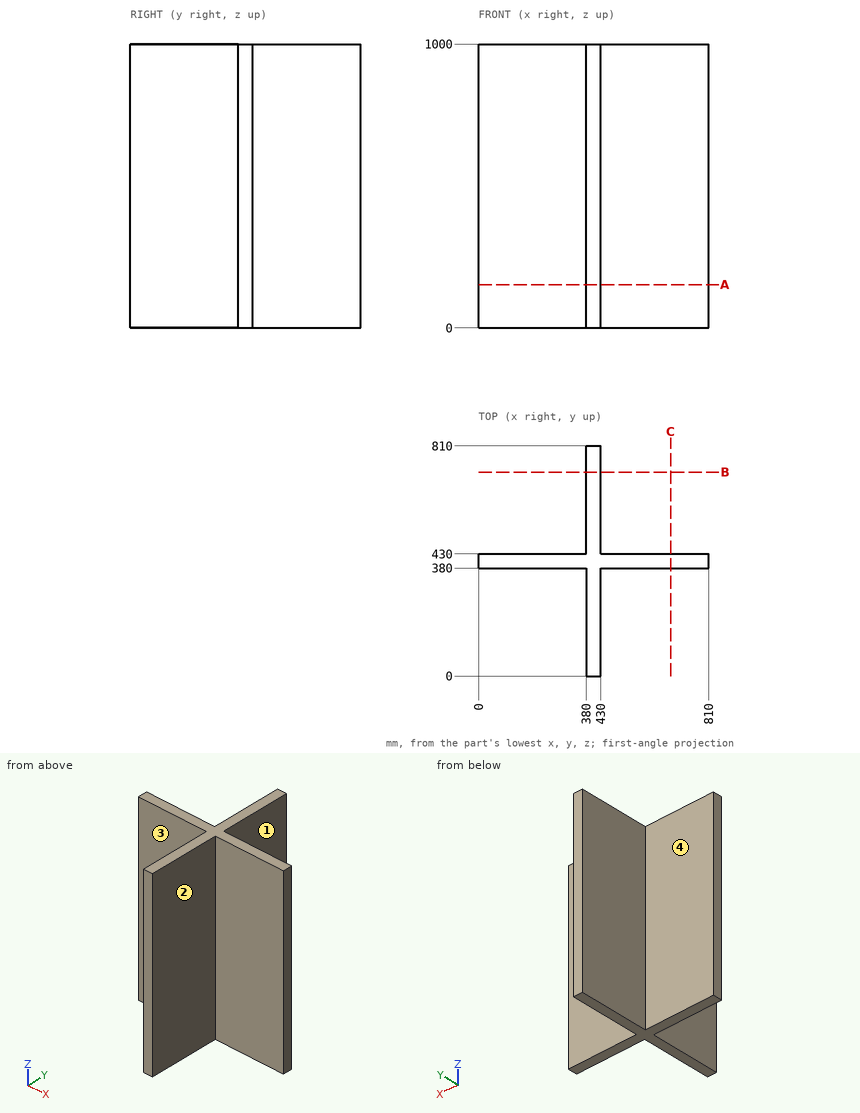
Geometry: see drawing. Coordinates: mm, zero at the bounding-box minimum. A direction names the side the tool comes from. Give positions to 0.01 mm unless a question says otherwise; leave off trailing zeros. Order: outer loops, then holes, each group sorted by start corner. A loop starts at its lowest first (then second) coordinate and runs counter-clockwise, first axis right, second up.
Q1. Contact query for flat-ended pins moving along their axis: pin 1 Ø6 at (x, z) = (525, 598) entering from +Y; pin 2 Ø1.5 at (y, z) = (270.5, 600) entering from +X; pin 3 Ø5 at (y, z) = (262, 652) entering from -X. Output: stop coordinate, or through.
Checked values:
pin 1: stops at y = 430
pin 2: stops at x = 430
pin 3: stops at x = 380
Q2. Section B-B on y = 718. Output: boundary loops of the cut face in (x, z).
Checked values:
outline: (380, 0) - (430, 0) - (430, 1000) - (380, 1000) - close
Q3. Set-up query: the marked faces 1, 2, 3 and 4. Return all of +Z, -Z, +X, -X, +Y, -Y with unobstructed straight access to the full face (end or side cutting, diameter ignored); none if empty.
Checked values:
face 1: +Z, -Z, +X, +Y
face 2: +Z, -Z, +X, -Y
face 3: +Z, -Z, -X, -Y
face 4: +Z, -Z, -X, +Y
Q4. Section A-A on z = 152.5. Output: boundary loops of the cut face in (x, y), and give its area (3 significant figures).
Checked values:
outline: (0, 380) - (380, 380) - (380, 0) - (430, 0) - (430, 380) - (810, 380) - (810, 430) - (430, 430) - (430, 810) - (380, 810) - (380, 430) - (0, 430) - close
area: 78,500 mm2
Q5. Ray query, probe 1 along Y at (x, z) = (631.5, 377.5). Return the intervals inside material, ascending.
Checked values:
probe 1: y = 380 to 430
